Here's how the part is built. I have some questions about the finished solid (model axes, mm). A direction names the side the tool comes from. Round coordinates to 2 decimals unless told otherwise and drop trailing zeros. Write each loop counter-clockwise with the first axis right and the second up, starting at its lowest first coordinate (ties: lowest second). Pieces come first, ordered by that corner, then holes. Notation, with made-up numbers: (36, 17) -> (40, 17) arc R24 cw to (40, 32) -> close; hole circle Ø10 at (-25, -15.75). An arc over 180 degrees is marked (long way). Put each result on its own line as item: value. Start each with the question number.
1. Which directions (+Z, -Z, +X, -X, +Y, -Y) give clear straight access to the entire face, cutting with the end or side of a thin tool? Please do faces 1 (the face through (0, 21.2, 13)), 2 (the face through (10, 0, 7)), 3 (the face through (10, -1.2, 3)), 4 (the face through (0, 23, 3.5)), 5 (the face through (18, 23.6, 5.7)).
2. Suppose I cut it at D-D (y = -8.5). Please give me the cut outline in (x, z), then the cut area to 3 significant figures.
3. We'd pull the mould along Z, two halves only. Please class faces 6 (the face through (0, 21.2, 2)), 7 (the face through (10, -10, 13.5)), 8 (the face through (0, 27.2, 7)), 9 (the face through (10, -8, 1.5)): +Z half, -Z half, draft (parallel to the pull), parting line (faces both ways), or undercut.
4. Suppose I cut it at A-A (z = 2.75). Please give me the cut outline in (x, y).
5. I need wall thicknesses on probe 1 along Z at (x, y) = (1.7, 24.2); probe 2 along Z at (x, y) = (16.5, -13) (3 decimals); probe 3 along Y at (x, z) = (14.25, 7.5). Which ranges of each line are inside material? Lowest first, please. Write a range as from..to.
6. Suppose I cut it at C-C (x = 16.75). Please give me the cut outline in (y, z).
7. Suppose I cut it at B-B (y = 1.5). Please give me the cut outline in (x, z).
8. For pin 1 (1.6 mm diameter, centred on x = 20, y = 23, fed in from +Z); pin 2 (5 mm diameter, centred on y = 24.5, z = 7.5, fed in from -X); pin 3 (0.6 mm diameter, centred on x = 1, z = 9.5, fed in from -Y), each with a flat end and sliding along its axis, tell me the tip position at first contact or that it passes through.
```python
from build123d import *

# Parameters (mm, degrees)
F1_DEPTH  = 15
F3_DEPTH  = 22.4
F5_DEPTH  = 25
F6_START  = -10
F6_DEPTH  = 15
F7_W      = 3.2
F7_H      = 8
F8_DEPTH  = 8
F9_R      = 3.99999
F10_R     = 1.5
F11_DEPTH = 25
F12_DEPTH = 2
F13_START = -20.4
F13_DEPTH = 4.6


# Not quite as in the source:
# - a fillet or chamfer is up to 0.001 mm smaller than in the source, because OpenCascade refuses the exact size


with BuildPart() as f1:
    # F0 (on Top) → F1 (new body)
    with BuildSketch(Plane.XY):
        Polygon((20, 0), (0, 0), (0, 20), (2, 20), (2, 21.2), (-1.2, 21.2), (-1.2, -1.2), (21.2, -1.2), (21.2, 21.2), (18, 21.2), (18, 20), (20, 20), align=None)
    extrude(amount=F1_DEPTH)

    # F2 (on face) → F3 (join)
    with BuildSketch(Plane(origin=(-1.2, 0, 0), x_dir=(0, -1, 0), z_dir=(-1, 0, 0))):
        with BuildLine():
            Line((1.2, 5.5), (7.5431457505, 5.5))
            ThreePointArc((7.5431457505, 5.5), (8.3010205144, 10.9641016151), (13.2, 13.5))
            Line((13.2, 13.5), (1.2, 13.5))
            Line((1.2, 13.5), (1.2, 5.5))
        make_face()
        with BuildLine():
            ThreePointArc((17.2, 7.5), (16.0284271247, 4.6715728753), (13.2, 3.5))
            Line((13.2, 3.5), (8.727864045, 3.5))
            ThreePointArc((8.727864045, 3.5), (10.7505102572, 2.0227744249), (13.2, 1.5))
            ThreePointArc((13.2, 1.5), (17.4426406871, 3.2573593129), (19.2, 7.5))
            ThreePointArc((19.2, 7.5), (17.4426406871, 11.7426406871), (13.2, 13.5))
            ThreePointArc((13.2, 13.5), (8.3010205144, 10.9641016151), (7.5431457505, 5.5))
            Line((7.5431457505, 5.5), (9.7358983849, 5.5))
            ThreePointArc((9.7358983849, 5.5), (12.1647238196, 11.3637033052), (17.2, 7.5))
        make_face()
        with BuildLine():
            ThreePointArc((13.2, 1.5), (10.7505102572, 2.0227744249), (8.727864045, 3.5))
            Line((8.727864045, 3.5), (2.727864045, 3.5))
            Line((2.727864045, 3.5), (2.727864045, 1.5))
            Line((2.727864045, 1.5), (13.2, 1.5))
        make_face()
    extrude(amount=-F3_DEPTH)

    # F4 (on face) → F5 (cut)
    with BuildSketch(Plane(origin=(0, 0, 1.5), x_dir=(1, 0, 0), z_dir=(0, 0, -1))):
        with BuildLine():
            ThreePointArc((8.5, 6.227864045), (8.9393398282, 5.1672038732), (10, 4.727864045))
            Line((10, 4.727864045), (10, 6.227864045))
            Line((10, 6.227864045), (8.5, 6.227864045))
        make_face()
        with BuildLine():
            Line((10, 6.227864045), (10, 4.727864045))
            ThreePointArc((10, 4.727864045), (11.0606601718, 5.1672038732), (11.5, 6.227864045))
            ThreePointArc((11.5, 6.227864045), (10, 7.727864045), (8.5, 6.227864045))
            Line((8.5, 6.227864045), (10, 6.227864045))
        make_face()
    extrude(amount=-F5_DEPTH, mode=Mode.SUBTRACT)

    # F4 (on face) → F6 (cut)
    with BuildSketch(Plane(origin=(0, 0, 1.5), x_dir=(1, 0, 0), z_dir=(0, 0, -1)).offset(F6_START)):
        with BuildLine():
            Line((10, 4.727864045), (10, 2.7637624299))
            Line((10, 2.7637624299), (13, 4.4958132374))
            Line((13, 4.4958132374), (13, 7.9599148526))
            Line((13, 7.9599148526), (10, 9.6919656601))
            Line((10, 9.6919656601), (7, 7.9599148526))
            Line((7, 7.9599148526), (7, 6.227864045))
            Line((7, 6.227864045), (8.5, 6.227864045))
            ThreePointArc((8.5, 6.227864045), (10, 7.727864045), (11.5, 6.227864045))
            ThreePointArc((11.5, 6.227864045), (11.0606601718, 5.1672038732), (10, 4.727864045))
        make_face()
        with BuildLine():
            Line((7, 4.4958132374), (10, 2.7637624299))
            Line((10, 2.7637624299), (10, 4.727864045))
            ThreePointArc((10, 4.727864045), (8.9393398282, 5.1672038732), (8.5, 6.227864045))
            Line((8.5, 6.227864045), (7, 6.227864045))
            Line((7, 6.227864045), (7, 4.4958132374))
        make_face()
    extrude(amount=-F6_DEPTH, mode=Mode.SUBTRACT)

    # F7 (on face) → F8 (join)
    with BuildSketch(Plane(origin=(0, 21.2, 0), x_dir=(-1, 0, 0), z_dir=(0, 1, 0))):
        with Locations((-19.6, 7.5)):
            Rectangle(F7_W, F7_H)
        with Locations((-0.4, 7.5)):
            Rectangle(F7_W, F7_H)
    extrude(amount=F8_DEPTH)

    # F9 (radius 4 in the source; OpenCascade refuses exactly that, so slightly less here)
    f9_edges = [f1.edges().sort_by_distance(p)[0] for p in [
        (19.6, 29.2, 11.5),
        (19.6, 29.2, 3.5),
        (0.4, 29.2, 11.5),
        (0.4, 29.2, 3.5),
    ]]
    fillet(f9_edges, radius=F9_R)

    # F10 (on face) → F11 (cut)
    with BuildSketch(Plane.YZ.offset(21.2)):
        with Locations((24.2, 7.5)):
            Circle(F10_R)
    extrude(amount=-F11_DEPTH, mode=Mode.SUBTRACT)

    # F10 (on face) → F12 (cut)
    with BuildSketch(Plane.YZ.offset(21.2)):
        with BuildLine():
            ThreePointArc((25.7000000635, 4.9019238253), (26.7980762297, 6.0000000317), (27.2, 7.5))
            ThreePointArc((27.2, 7.5), (26.7980761988, 9.0000000218), (25.6999999564, 10.0980762365))
            ThreePointArc((25.6999999564, 10.0980762365), (24.2, 10.5), (22.7000000436, 10.0980762365))
            ThreePointArc((22.7000000436, 10.0980762365), (21.6019238012, 9.0000000218), (21.2, 7.5))
            ThreePointArc((21.2, 7.5), (21.6019238012, 5.9999999782), (22.7000000436, 4.9019237635))
            ThreePointArc((22.7000000436, 4.9019237635), (24.2000000618, 4.5), (25.7000000635, 4.9019238253))
        make_face()
        with Locations((24.2, 7.5)):
            Circle(F10_R, mode=Mode.SUBTRACT)
    extrude(amount=-F12_DEPTH, mode=Mode.SUBTRACT)

    # F10 (on face) → F13 (cut)
    with BuildSketch(Plane.YZ.offset(21.2).offset(F13_START)):
        with BuildLine():
            ThreePointArc((21.2, 7.5), (21.6019238012, 9.0000000218), (22.7000000436, 10.0980762365))
            Line((22.7000000436, 10.0980762365), (21.2, 9.2320508076))
            Line((21.2, 9.2320508076), (21.2, 7.5))
        make_face()
        with BuildLine():
            ThreePointArc((22.7000000436, 10.0980762365), (24.2, 10.5), (25.6999999564, 10.0980762365))
            Line((25.6999999564, 10.0980762365), (24.2, 10.9641016151))
            Line((24.2, 10.9641016151), (22.7000000436, 10.0980762365))
        make_face()
        with BuildLine():
            ThreePointArc((25.6999999564, 10.0980762365), (26.7980761988, 9.0000000218), (27.2, 7.5))
            Line((27.2, 7.5), (27.2, 9.2320508076))
            Line((27.2, 9.2320508076), (25.6999999564, 10.0980762365))
        make_face()
        with BuildLine():
            ThreePointArc((25.7000000635, 4.9019238253), (26.7980762297, 6.0000000317), (27.2, 7.5))
            ThreePointArc((27.2, 7.5), (26.7980761988, 9.0000000218), (25.6999999564, 10.0980762365))
            ThreePointArc((25.6999999564, 10.0980762365), (24.2, 10.5), (22.7000000436, 10.0980762365))
            ThreePointArc((22.7000000436, 10.0980762365), (21.6019238012, 9.0000000218), (21.2, 7.5))
            ThreePointArc((21.2, 7.5), (21.6019238012, 5.9999999782), (22.7000000436, 4.9019237635))
            ThreePointArc((22.7000000436, 4.9019237635), (24.2000000618, 4.5), (25.7000000635, 4.9019238253))
        make_face()
        with Locations((24.2, 7.5)):
            Circle(F10_R, mode=Mode.SUBTRACT)
        with BuildLine():
            Line((24.2, 4.0358983849), (25.7000000635, 4.9019238253))
            ThreePointArc((25.7000000635, 4.9019238253), (24.2000000618, 4.5), (22.7000000436, 4.9019237635))
            Line((22.7000000436, 4.9019237635), (24.2, 4.0358983849))
        make_face()
        with BuildLine():
            Line((21.2, 5.7679491924), (22.7000000436, 4.9019237635))
            ThreePointArc((22.7000000436, 4.9019237635), (21.6019238012, 5.9999999782), (21.2, 7.5))
            Line((21.2, 7.5), (21.2, 5.7679491924))
        make_face()
        with BuildLine():
            Line((27.2, 5.7679491924), (27.2, 7.5))
            ThreePointArc((27.2, 7.5), (26.7980762297, 6.0000000317), (25.7000000635, 4.9019238253))
            Line((25.7000000635, 4.9019238253), (27.2, 5.7679491924))
        make_face()
    extrude(amount=-F13_DEPTH, mode=Mode.SUBTRACT)


solid = f1.part
```
Verdict:
1. face 1: +Z, +X, -X, +Y
1. face 2: +Z, -Z
1. face 3: -Z, +X, -X
1. face 4: -Z, +X, -X, +Y
1. face 5: +Z, -Z, +Y
2. outline: (-1.2, 1.5) -> (21.2, 1.5) -> (21.2, 3.5) -> (-1.2, 3.5) -> close; (-1.2, 5.5) -> (21.2, 5.5) -> (21.2, 13.5) -> (12.06, 13.5) -> (12.06, 11.5) -> (7.94, 11.5) -> (7.94, 13.5) -> (-1.2, 13.5) -> close
2. area: 216 mm^2
3. face 6: draft
3. face 7: +Z half
3. face 8: undercut
3. face 9: -Z half
4. outline: (-1.2, -16.87) -> (21.2, -16.87) -> (21.2, -2.73) -> (-1.2, -2.73) -> close; (-1.2, -1.2) -> (21.2, -1.2) -> (21.2, 21.2) -> (18, 21.2) -> (18, 20) -> (20, 20) -> (20, 0) -> (0, 0) -> (0, 20) -> (2, 20) -> (2, 21.2) -> (-1.2, 21.2) -> close; hole circle Ø3 at (10, -6.23)
5. probe 1: z = 3.5..6, 9..11.5
5. probe 2: z = 1.5..3.5, 11.495..13.5
5. probe 3: y = -19.2..-17.2, -9.2..0
6. outline: (-13.2, 1.5) -> (-2.73, 1.5) -> (-2.73, 3.5) -> (-13.2, 3.5) arc R4 cw (long way) to (-9.74, 5.5) -> (-1.2, 5.5) -> (-1.2, 0) -> (0, 0) -> (0, 15) -> (-1.2, 15) -> (-1.2, 13.5) -> (-13.2, 13.5) arc R6 ccw to start
7. outline: (-1.2, 0) -> (0, 0) -> (0, 15) -> (-1.2, 15) -> close; (20, 0) -> (21.2, 0) -> (21.2, 15) -> (20, 15) -> close
8. pin 1: stops at z = 11.5
8. pin 2: stops at x = 0.8
8. pin 3: stops at y = -18.95
